```python
from build123d import *

# Parameters (mm, degrees)
SKETCH1_W                        = 210
SKETCH1_H                        = 45
BASE_FLANGE1_DEPTH               = 2
SM_EDGE_FLANGE_1_STRIP_W         = 12
SM_EDGE_FLANGE_1_STRIP_H         = 2
SM_EDGE_FLANGE_1_STRIP_CUT_DEPTH = 210
SM_EDGE_FLANGE_1_DEPTH           = 210
CUT_EXTRUDE1_START               = -86.312353883
CUT_EXTRUDE1_DEPTH               = 181.312353883
CUT_EXTRUDE1_START_2             = -95
CUT_EXTRUDE1_2_DEPTH             = 8.687646117


# Read off the part's stored shape, not the designer's step: Cut-Extrude1
# Sheet-metal steps are written as plain solids
with BuildPart() as part:
    # Sketch1 → Base-Flange1 (new body)
    with BuildSketch(Plane.XY):
        Rectangle(SKETCH1_W, SKETCH1_H)
    extrude(amount=-BASE_FLANGE1_DEPTH)

    # Ребро-кромка1 strip (across the edge) → Ребро-кромка1 strip cut (cut)
    with BuildSketch(Plane(origin=(-105, -22.5, 0), x_dir=(0, 1, 0), z_dir=(1, 0, 0))):
        with Locations((-2, -1)):
            Rectangle(SM_EDGE_FLANGE_1_STRIP_W, SM_EDGE_FLANGE_1_STRIP_H)
    extrude(amount=SM_EDGE_FLANGE_1_STRIP_CUT_DEPTH, mode=Mode.SUBTRACT)

    # Ребро-кромка1 section (across the edge) → Ребро-кромка1 (add)
    with BuildSketch(Plane(origin=(-105, -22.5, 0), x_dir=(0, 1, 0), z_dir=(1, 0, 0))):
        with BuildLine():
            Line((0, 2), (0, 23))
            Line((0, 23), (2, 23))
            Line((2, 23), (2, 2))
            ThreePointArc((2, 2), (2.585786438, 0.585786438), (4, 0))
            Line((4, 0), (4, -2))
            ThreePointArc((4, -2), (1.171572875, -0.828427125), (0, 2))
        make_face()
    extrude(amount=SM_EDGE_FLANGE_1_DEPTH)

    # Cut-Extrude1 outline → Cut-Extrude1 (cut)
    with BuildSketch(Plane.YZ.offset(CUT_EXTRUDE1_START)):
        with BuildLine():
            Line((-20.5, 2), (-20.5, 23))
            Line((-20.5, 23), (-22.5, 23))
            Line((-22.5, 23), (-22.5, 2))
            ThreePointArc((-22.5, 2), (-21.964101615, 0), (-20.5, -1.464101615))
            Line((-20.5, -1.464101615), (-19.5, 0.267949193))
            ThreePointArc((-19.5, 0.267949193), (-20.232050807, 1), (-20.5, 2))
        make_face()
    extrude(amount=CUT_EXTRUDE1_DEPTH, mode=Mode.SUBTRACT)

    # Cut-Extrude1 2 outline → Cut-Extrude1 2 (cut)
    with BuildSketch(Plane.YZ.offset(CUT_EXTRUDE1_START_2)):
        with BuildLine():
            Line((-20.5, 2), (-20.5, 14.70719641))
            Line((-20.5, 14.70719641), (-22.5, 14.70719641))
            Line((-22.5, 14.70719641), (-22.5, 2))
            ThreePointArc((-22.5, 2), (-21.964101615, 0), (-20.5, -1.464101615))
            Line((-20.5, -1.464101615), (-19.5, 0.267949193))
            ThreePointArc((-19.5, 0.267949193), (-20.232050807, 1), (-20.5, 2))
        make_face()
    extrude(amount=CUT_EXTRUDE1_2_DEPTH, mode=Mode.SUBTRACT)


solid = part.part
```
Check sheet for the modelled part. Datum: model origin and axes. Units: mm. A direction names the side the tool comes from. Round coordinates to 2 decimals unless told otherwise and drop trailing zeros. Loops run counter-clockwise (first coordinate to the right, second up) from the corner with the lowest first, then second, coordinate; pieces in that order, holes last. Notation, with made-up numbers: (-3.75, 78.5) - (10.25, 78.5) arc R27 cw to (10.25, 98.5) - close; hole circle Ø10 at (-8, -4.75). An arc over 180 degrees is marked (long way). Write item = value, one per line. Start each with the question number.
Q1. Thickness scan on L1, parallel to Z at x = 21, y = -14. Record the ranges inside material, lowest first.
Q2. Section check C-C (x = -12). Record the boundary of the cut face in (y, z).
Q3. Depth check by flat-ended pin: P1, Ø3, axis at x = 100, z = 14, coming from the +Y side; P2, Ø1, axis at x = -91.5, y = -21.5, coming from the -Z side; P3, Ø10, axis at x = -54, y = 8, coming from the +Z side. Enter the tip coordinate at first touch or a pass-through.
Q4. Release check for a two-part mould opening along Z. For faces 1 (the face through (-1, 2, 0)), 2 (the face through (100, -20.5, 13)), 3 (the face through (-1, 2, -2)) record: pulls with the +Z half, pulls with the -Z half, needs draft (parallel to the pull), parting line crosses it, or undercut.
Q5. Access from +Z, -Z, +X, -X, +Y, -Y to the whole of each face (thin tool, end or side, straight path). Record for faces 4 (the face through (-98, -20.5, 15)), 5 (the face through (105, -7, -1)).
Q6. Section check D-D (y = -9). Record the boundary of the cut face in (x, z).
Q7. Section check B-B (z = 18.75). Record the boundary of the cut face in (x, y), plus the area to 3 significant figures.
Q8. Section check A-A (z = 6.5). Record the boundary of the cut face in (x, y).
Derived:
q1.L1 = -2 to 0
q2.outline = (-20.5, -1.46) arc R4 ccw to (-18.5, -2) - (22.5, -2) - (22.5, 0) - (-18.5, 0) arc R2 cw to (-19.5, 0.27) - close
q3.P1 = -20.5
q3.P2 = 14.71
q3.P3 = 0
q4.face_1 = pulls with the +Z half
q4.face_2 = needs draft
q4.face_3 = pulls with the -Z half
q5.face_4 = +Z, +X, -X, +Y
q5.face_5 = +Z, -Z, +X, +Y, -Y
q6.outline = (-105, -2) - (105, -2) - (105, 0) - (-105, 0) - close
q7.outline = (-105, -22.5) - (-86.31, -22.5) - (-86.31, -20.5) - (-105, -20.5) - close; (95, -22.5) - (105, -22.5) - (105, -20.5) - (95, -20.5) - close
q7.area = 57.4 mm^2
q8.outline = (-105, -22.5) - (-95, -22.5) - (-95, -20.5) - (-105, -20.5) - close; (95, -22.5) - (105, -22.5) - (105, -20.5) - (95, -20.5) - close
